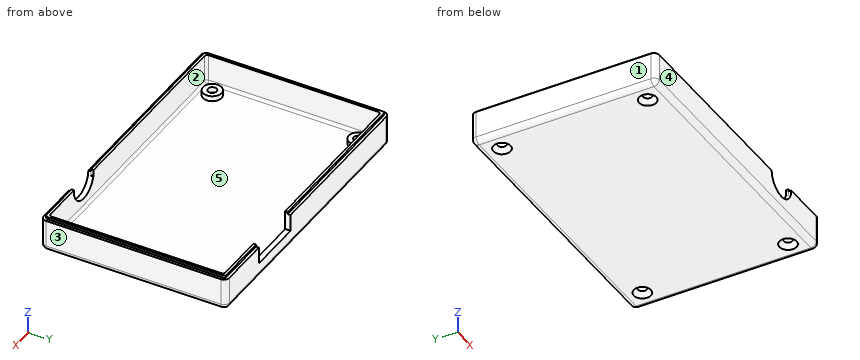
```python
from build123d import *

# Parameters (mm, degrees)
F0_W           = 104
F0_H           = 66
F0_R           = 3
F1_DEPTH       = 2
F2_DEPTH       = 10.99
F3_DEPTH       = 10.1
F4_R           = 3.5
F5_DEPTH       = 2
F7_D           = 3.302
F7_CSINK_D     = 6.477
F7_CSINK_ANGLE = 82
F8_W           = 21
F8_H           = 6.4
F9_DEPTH       = 2.5
F10_W          = 13
F10_H          = 0.95
F11_DEPTH      = 2.5
F13_DEPTH      = 2.5
F14_R          = 2
F15_R          = 1
F16_W          = 21
F16_H          = 0.89
F17_DEPTH      = 2.5


# Not quite as in the source:
# - a feature names something its author has since deleted; it is built from what else it names


with BuildPart() as f1:
    # F0 (on Top) → F1 (new body)
    with BuildSketch(Plane.XY):
        with BuildLine():
            Line((61.6408709802, 21.8759292028), (-42.3591290198, 21.8759292028))
            ThreePointArc((-42.3591290198, 21.8759292028), (-43.7733425821, 21.2901427652), (-44.3591290198, 19.8759292028))
            Line((-44.3591290198, 19.8759292028), (-44.3591290198, -46.1240707972))
            ThreePointArc((-44.3591290198, -46.1240707972), (-43.7733425821, -47.5382843595), (-42.3591290198, -48.1240707972))
            Line((-42.3591290198, -48.1240707972), (61.6408709802, -48.1240707972))
            ThreePointArc((61.6408709802, -48.1240707972), (63.0550845426, -47.5382843595), (63.6408709802, -46.1240707972))
            Line((63.6408709802, -46.1240707972), (63.6408709802, 19.8759292028))
            ThreePointArc((63.6408709802, 19.8759292028), (63.0550845426, 21.2901427652), (61.6408709802, 21.8759292028))
        make_face()
        with BuildLine():
            ThreePointArc((-43.3091290198, 19.8759292028), (-43.0308804619, 20.547680645), (-42.3591290198, 20.8259292028))
            Line((-42.3591290198, 20.8259292028), (61.6408709802, 20.8259292028))
            ThreePointArc((61.6408709802, 20.8259292028), (62.3126224224, 20.547680645), (62.5908709802, 19.8759292028))
            Line((62.5908709802, 19.8759292028), (62.5908709802, -46.1240707972))
            ThreePointArc((62.5908709802, -46.1240707972), (62.3126224224, -46.7958222393), (61.6408709802, -47.0740707972))
            Line((61.6408709802, -47.0740707972), (-42.3591290198, -47.0740707972))
            ThreePointArc((-42.3591290198, -47.0740707972), (-43.0308804619, -46.7958222393), (-43.3091290198, -46.1240707972))
            Line((-43.3091290198, -46.1240707972), (-43.3091290198, 19.8759292028))
        make_face(mode=Mode.SUBTRACT)
        with BuildLine():
            Line((61.6408709802, 20.8259292028), (-42.3591290198, 20.8259292028))
            ThreePointArc((-42.3591290198, 20.8259292028), (-43.0308804619, 20.547680645), (-43.3091290198, 19.8759292028))
            Line((-43.3091290198, 19.8759292028), (-43.3091290198, -46.1240707972))
            ThreePointArc((-43.3091290198, -46.1240707972), (-43.0308804619, -46.7958222393), (-42.3591290198, -47.0740707972))
            Line((-42.3591290198, -47.0740707972), (61.6408709802, -47.0740707972))
            ThreePointArc((61.6408709802, -47.0740707972), (62.3126224224, -46.7958222393), (62.5908709802, -46.1240707972))
            Line((62.5908709802, -46.1240707972), (62.5908709802, 19.8759292028))
            ThreePointArc((62.5908709802, 19.8759292028), (62.3126224224, 20.547680645), (61.6408709802, 20.8259292028))
        make_face()
        with Locations((9.6408709802, -13.1240707972)):
            Rectangle(F0_W, F0_H, mode=Mode.SUBTRACT)
        with Locations((9.6408709802, -13.1240707972)):
            Rectangle(F0_W, F0_H)
        with Locations((-36.8591290198, -40.6240707972)):
            Circle(F0_R, mode=Mode.SUBTRACT)
        with Locations((57.1408709802, -40.6240707972)):
            Circle(F0_R, mode=Mode.SUBTRACT)
        with Locations((-36.8591290198, 14.3759292028)):
            Circle(F0_R, mode=Mode.SUBTRACT)
        with Locations((57.1408709802, 14.3759292028)):
            Circle(F0_R, mode=Mode.SUBTRACT)
        with Locations((-36.8591290198, -40.6240707972)):
            Circle(F0_R)
        with Locations((57.1408709802, -40.6240707972)):
            Circle(F0_R)
        with Locations((-36.8591290198, 14.3759292028)):
            Circle(F0_R)
        with Locations((57.1408709802, 14.3759292028)):
            Circle(F0_R)
    extrude(amount=-F1_DEPTH)

    # F0 (on Top) → F2 (join)
    with BuildSketch(Plane.XY):
        with BuildLine():
            Line((61.6408709802, 20.8259292028), (-42.3591290198, 20.8259292028))
            ThreePointArc((-42.3591290198, 20.8259292028), (-43.0308804619, 20.547680645), (-43.3091290198, 19.8759292028))
            Line((-43.3091290198, 19.8759292028), (-43.3091290198, -46.1240707972))
            ThreePointArc((-43.3091290198, -46.1240707972), (-43.0308804619, -46.7958222393), (-42.3591290198, -47.0740707972))
            Line((-42.3591290198, -47.0740707972), (61.6408709802, -47.0740707972))
            ThreePointArc((61.6408709802, -47.0740707972), (62.3126224224, -46.7958222393), (62.5908709802, -46.1240707972))
            Line((62.5908709802, -46.1240707972), (62.5908709802, 19.8759292028))
            ThreePointArc((62.5908709802, 19.8759292028), (62.3126224224, 20.547680645), (61.6408709802, 20.8259292028))
        make_face()
        with Locations((9.6408709802, -13.1240707972)):
            Rectangle(F0_W, F0_H, mode=Mode.SUBTRACT)
    extrude(amount=F2_DEPTH)

    # F0 (on Top) → F3 (join)
    with BuildSketch(Plane.XY):
        with BuildLine():
            Line((61.6408709802, 21.8759292028), (-42.3591290198, 21.8759292028))
            ThreePointArc((-42.3591290198, 21.8759292028), (-43.7733425821, 21.2901427652), (-44.3591290198, 19.8759292028))
            Line((-44.3591290198, 19.8759292028), (-44.3591290198, -46.1240707972))
            ThreePointArc((-44.3591290198, -46.1240707972), (-43.7733425821, -47.5382843595), (-42.3591290198, -48.1240707972))
            Line((-42.3591290198, -48.1240707972), (61.6408709802, -48.1240707972))
            ThreePointArc((61.6408709802, -48.1240707972), (63.0550845426, -47.5382843595), (63.6408709802, -46.1240707972))
            Line((63.6408709802, -46.1240707972), (63.6408709802, 19.8759292028))
            ThreePointArc((63.6408709802, 19.8759292028), (63.0550845426, 21.2901427652), (61.6408709802, 21.8759292028))
        make_face()
        with BuildLine():
            ThreePointArc((-43.3091290198, 19.8759292028), (-43.0308804619, 20.547680645), (-42.3591290198, 20.8259292028))
            Line((-42.3591290198, 20.8259292028), (61.6408709802, 20.8259292028))
            ThreePointArc((61.6408709802, 20.8259292028), (62.3126224224, 20.547680645), (62.5908709802, 19.8759292028))
            Line((62.5908709802, 19.8759292028), (62.5908709802, -46.1240707972))
            ThreePointArc((62.5908709802, -46.1240707972), (62.3126224224, -46.7958222393), (61.6408709802, -47.0740707972))
            Line((61.6408709802, -47.0740707972), (-42.3591290198, -47.0740707972))
            ThreePointArc((-42.3591290198, -47.0740707972), (-43.0308804619, -46.7958222393), (-43.3091290198, -46.1240707972))
            Line((-43.3091290198, -46.1240707972), (-43.3091290198, 19.8759292028))
        make_face(mode=Mode.SUBTRACT)
    extrude(amount=F3_DEPTH)

    # F4 (on face) → F5 (join)
    with BuildSketch(Plane.XY):
        with Locations((-36.8591290198, 14.3759292028)):
            Circle(F4_R)
        with Locations((56.1408709802, 14.3759292028)):
            Circle(F4_R)
        with Locations((56.1408709802, -40.6240707972)):
            Circle(F4_R)
        with Locations((-36.8591290198, -40.6240707972)):
            Circle(F4_R)
    extrude(amount=F5_DEPTH)

    # F7 (through all)
    with Locations(Plane(origin=(0, 0, -2), x_dir=(1, 0, 0), z_dir=(0, 0, -1))):
        with Locations((-36.8591290198, 40.6240707972), (56.1408709802, 40.6240707972), (56.1408709802, -14.3759292028), (-36.8591290198, -14.3759292028)):
            CounterSinkHole(F7_D / 2, F7_CSINK_D / 2, counter_sink_angle=F7_CSINK_ANGLE)

    # F8 (on face) → F9 (cut)
    with BuildSketch(Plane(origin=(0, 21.8759292028, 0), x_dir=(-1, 0, 0), z_dir=(0, 1, 0))):
        with Locations((-31.5408709802, 6.9)):
            Rectangle(F8_W, F8_H)
    extrude(amount=-F9_DEPTH, mode=Mode.SUBTRACT)

    # F10 (on face) → F11 (cut)
    with BuildSketch(Plane.XY.offset(10.99)):
        with Locations((38.6408709802, -46.5990707972)):
            Rectangle(F10_W, F10_H)
    extrude(amount=-F11_DEPTH, mode=Mode.SUBTRACT)

    # F12 (on face) → F13 (cut)
    with BuildSketch(Plane.XZ.offset(48.1240707972)):
        with BuildLine():
            ThreePointArc((32.1408709802, 10.1), (38.6408709802, 3.6), (45.1408709802, 10.1))
            Line((45.1408709802, 10.1), (32.1408709802, 10.1))
        make_face()
    extrude(amount=-F13_DEPTH, mode=Mode.SUBTRACT)

    # F14
    f14_edges = [f1.edges().sort_by_distance(p)[0] for p in [
        (63.640871, -13.124071, -2),
        (9.640871, 21.875929, -2),
        (-44.359129, -13.124071, -2),
        (9.640871, -48.124071, -2),
        (63.055085, 21.290143, -2),
        (-43.773343, 21.290143, -2),
        (63.055085, -47.538284, -2),
        (-43.773343, -47.538284, -2),
    ]]
    fillet(f14_edges, radius=F14_R)

    # F15
    f15_edges = [f1.edges().sort_by_distance(p)[0] for p in [
        (9.640871, 19.875929, 0),
        (-42.359129, 19.875929, 5.495),
        (-42.359129, -13.124071, 0),
        (9.640871, -46.124071, 0),
        (-42.359129, -46.124071, 5.495),
        (61.640871, 19.875929, 5.495),
        (61.640871, -13.124071, 0),
        (61.640871, -46.124071, 5.495),
    ]]
    fillet(f15_edges, radius=F15_R)

    # F16 (on face) → F17 (cut)
    with BuildSketch(Plane(origin=(0, 20.8259292028, 0), x_dir=(-1, 0, 0), z_dir=(0, 1, 0))):
        with Locations((-31.5408709802, 10.545)):
            Rectangle(F16_W, F16_H)
    extrude(amount=-F17_DEPTH, mode=Mode.SUBTRACT)


solid = f1.part
```
Here's how the part is built. I have some questions about the finished solid (model axes, mm). Face numbers are marked on the shaded views. A direction names the side the tool comes from. Round coordinates to 2 decimals unless told otherwise and drop trailing zeros. Order: outer loops, then holes, each group sorted by start corner. A loop starts at its lowest first (then second) coordinate and runs counter-clockwise, first axis right, second up. Notation, with made-up numbers: M 72.5,14.25 L 115.5,14.25 A8 ccw 115.5,23.25 Z; hole C 1,89 d2. An arc over 180 degrees is marked long. Answer as CSV lines item,"result".
Item 1: Imagine slicing it at A-A on x = -15.5. List the corners of the cut face in (y, z) for me, and give its area (3 significant figures).
From the geometry:
outline,"M -48.12,0 A2 ccw -46.12,-2 L 19.88,-2 A2 ccw 21.88,0 L 21.88,10.1 L 20.83,10.1 L 20.83,10.99 L 19.88,10.99 L 19.88,1 A1 cw 18.88,0 L -45.12,0 A1 cw -46.12,1 L -46.12,10.99 L -47.07,10.99 L -47.07,10.1 L -48.12,10.1 Z"
area,"181 mm2"
Item 2: Which directions (+Z, -Z, +X, -X, +Y, -Y) give clear straight access to the entire face, cutting with the end or side of a thin tool? Please do the marked faces 4 and 5.
From the geometry:
face 4,"+Z, -Z, +X, -X, -Y"
face 5,"+Z"
Item 3: For pin 1 (0.7 mm diameter, centred on x = 47, z = 10.5, fed in from +Y); pin 2 (8 mm diameter, centred on x = -11.5, y = -8, fed in from +Z); pin 3 (7.5 mm diameter, centred on x = 56, y = 16, fed in from +Z); pin 4 (2 mm diameter, centred on x = -36.86, y = -40.62, fed in from +Z), each with a flat end and sliding along its axis, tell me the tip position at first contact or that it passes through.
From the geometry:
pin 1,"y = 20.83"
pin 2,"z = 0"
pin 3,"z = 2"
pin 4,"through"
Item 4: Imagine slicing it at B-B on z = 7. List the corners of the cut face in (x, y) for me, and give its area (3 significant figures).
From the geometry:
outline,"M -44.36,-46.12 A2 ccw -42.36,-48.12 L 32.93,-48.12 L 32.93,-46.12 L -41.36,-46.12 A1 cw -42.36,-45.12 L -42.36,18.88 A1 cw -41.36,19.88 L 21.04,19.88 L 21.04,21.88 L -42.36,21.88 A2 ccw -44.36,19.88 Z; M 42.04,19.88 L 60.64,19.88 A1 cw 61.64,18.88 L 61.64,-45.12 A1 cw 60.64,-46.12 L 44.35,-46.12 L 44.35,-48.12 L 61.64,-48.12 A2 ccw 63.64,-46.12 L 63.64,19.88 A2 ccw 61.64,21.88 L 42.04,21.88 Z"
area,"629 mm2"
Item 5: We'd pull the mould along X, two halves only. Please class the marked faces 1, 2 and 3: +X half, -X half, draft (parallel to the pull), parting line (faces both ways), or undercut.
From the geometry:
face 1,"-X half"
face 2,"undercut"
face 3,"+X half"
Item 6: Imagine slicing it at D-D on x = 40. List the corners of the cut face in (y, z) for me, and give its area (3 significant figures).
From the geometry:
outline,"M -48.12,0 A2 ccw -46.12,-2 L 19.88,-2 A2 ccw 21.88,0 L 21.88,3.7 L 19.88,3.7 L 19.88,1 A1 cw 18.88,0 L -45.12,0 A1 cw -46.12,1 L -46.12,3.74 L -48.12,3.74 Z"
area,"154 mm2"
Item 7: Imagine slicing it at C-C on y = -25. List the corners of the cut face in (x, z) for me, and give its area (3 significant figures).
From the geometry:
outline,"M -44.36,0 A2 ccw -42.36,-2 L 61.64,-2 A2 ccw 63.64,0 L 63.64,10.1 L 62.59,10.1 L 62.59,10.99 L 61.64,10.99 L 61.64,1 A1 cw 60.64,0 L -41.36,0 A1 cw -42.36,1 L -42.36,10.99 L -43.31,10.99 L -43.31,10.1 L -44.36,10.1 Z"
area,"257 mm2"
Item 8: Please list where these lines run through material, in increasing order: L1, parallel to X at y = -6, z = 1; L2, parallel to Y at x = 23.5, z = 2; L3, parallel to X at y = 14, z = 0.75. Write a range as [from, to].
From the geometry:
L1,"[-44.36, -42.36], [61.64, 63.64]"
L2,"[-48.12, -46.12], [19.88, 21.88]"
L3,"[-44.36, -42.33], [-40.34, -38.47], [-35.25, -33.38], [52.66, 54.53], [57.75, 59.62], [61.61, 63.64]"
